CAD build for the part. Positions are in the model's coordinates, mm. A direction names the side the tool comes from. Coordinates: 2 decimals unless noted, no trailing zeros. Loops run counter-clockwise (first coordinate to the right, second up) from the corner with the lowest first, then second, coordinate; pieces in that order, holes last. Notation, with made-up numbers: (12, -22) -> (42, -22) arc R14 ccw to (42, -3) -> close; hole circle Ø11 at (-37.75, 87). An arc over 180 degrees is marked (long way). Answer as CSV lines item,"result". Start each with the question number.
```python
from build123d import *

# Parameters (mm, degrees)
ESBO_O1_R                                   = 9.1
RESSALTO_EXTRUS_O1_DEPTH                    = 3
ESBO_O2_R                                   = 6.7
RESSALTO_EXTRUS_O2_DEPTH                    = 87
FURO_ROSCADO_PARA_CONDU_TE_DE_M4X0_72_D     = 4.2
FURO_ROSCADO_PARA_CONDU_TE_DE_M4X0_72_DEPTH = 22
FURO_ROSCADO_PARA_CONDU_TE_DE_M4X0_72_TIP   = 1.2618073
RESSALTO_EXTRUS_O3_DEPTH                    = 4


with BuildPart() as part:
    # Esboço1 → Ressalto-extrusão1 (new body)
    with BuildSketch(Plane.XY):
        Circle(ESBO_O1_R)
    extrude(amount=-RESSALTO_EXTRUS_O1_DEPTH)

    # Esboço2 → Ressalto-extrusão2 (add)
    with BuildSketch(Plane(origin=(0, 0, -3), x_dir=(-1, 0, 0), z_dir=(0, 0, -1))):
        Circle(ESBO_O2_R)
    extrude(amount=RESSALTO_EXTRUS_O2_DEPTH)

    # Furo roscado para conduíte de M4x0.72
    with Locations(Plane(origin=(0, 0, -90), x_dir=(-1, 0, 0), z_dir=(0, 0, -1))):
        with Locations((0, 0)):
            Hole(FURO_ROSCADO_PARA_CONDU_TE_DE_M4X0_72_D / 2, depth=FURO_ROSCADO_PARA_CONDU_TE_DE_M4X0_72_DEPTH)
            with Locations((0, 0, -(FURO_ROSCADO_PARA_CONDU_TE_DE_M4X0_72_DEPTH + FURO_ROSCADO_PARA_CONDU_TE_DE_M4X0_72_TIP / 2))):  # 118° drill point
                Cone(0, FURO_ROSCADO_PARA_CONDU_TE_DE_M4X0_72_D / 2, FURO_ROSCADO_PARA_CONDU_TE_DE_M4X0_72_TIP, mode=Mode.SUBTRACT)

    # Esboço7 → Ressalto-extrusão3 (add)
    with BuildSketch(Plane(origin=(0, 0, -90), x_dir=(-1, 0, 0), z_dir=(0, 0, -1))):
        with BuildLine():
            Line((-5.37494186, 4), (5.37494186, 4))
            ThreePointArc((5.37494186, 4), (0, 6.7), (-5.37494186, 4))
        make_face()
    extrude(amount=RESSALTO_EXTRUS_O3_DEPTH)


solid = part.part
```
Q1. Probe probe 1 along X at (y, z) = (0, -73.5); probe 2 along Z at (x, y) = (3.5, 6). List the from-to ranges inside material, lowest first. Write a range as from..to.
Q2. Saw through at C-C (z = -41). List the corners of the cut face in (x, y).
Q3. Two-plate mould, pull along Y, no slides. Class faces 4 (the flat face through (0, 5, -94)), 5 (the cylindrical face through (2.003, 0.631, -78.846)), 6 (the flat face through (0, 4, -92)), 7 (the conical face through (-0.35, 0.11, -66.96)): pulls with the +Y half, pulls with the -Y half, needs draft (parallel to the pull), parting line crosses it, or undercut.
Q4. Saw through at A-A (z = -83.5). List the corners of the cut face in (x, y), and give its area (3 significant figures).
Q5. Which spindle directions (+Z, -Z, +X, -X, +Y, -Y) get a long thin tool onto all of the face, cutting with end or side? Do faces 1 (the cylindrical face through (-1.973, -8.884, -1.479)), 2 (the flat face through (-1, -7, -3)), 3 (the flat face through (0.1, -2.5, -90)). Say none if no direction does.
Q6. Pin check, flat tips, straight feed: pin 1 Ø1 at (x, y) = (-3, 4.5) entering from +Z; pin 2 Ø4.5 at (x, z) = (0, -92) entering from -Y; pin 3 Ø3 at (x, z) = (-0.5, -33) entering from +Y; pin 4 Ø9 at (x, y) = (3, -4.5) entering from -Z. Stop position of each tip, or through.
Q7. Saw through at D-D (y = 5.5). List the corners of the cut face in (x, z), and give its area (3 significant figures).
Q8. Saw through at B-B (y = -4.75). List the corners of the cut face in (x, z), and give its area (3 significant figures).
Ans:
1,probe 1,"x = -6.7..-2.1, 2.1..6.7"
1,probe 2,"z = -3..0"
2,outline,"circle Ø13.4 at (0, 0)"
3,face 4,"needs draft"
3,face 5,"undercut"
3,face 6,"pulls with the -Y half"
3,face 7,"undercut"
4,outline,"circle Ø13.4 at (0, 0); hole circle Ø4.2 at (0, 0)"
4,area,"127 mm²"
5,face 1,"+Z, -Z"
5,face 2,"-Z"
5,face 3,"-Z, +X, -X, -Y"
6,pin 1,"stops at z = 0"
6,pin 2,"stops at y = -6.7"
6,pin 3,"stops at y = 6.7"
6,pin 4,"stops at z = -90"
7,outline,"(-7.25, -3) -> (-3.83, -3) -> (-3.83, -94) -> (3.83, -94) -> (3.83, -3) -> (7.25, -3) -> (7.25, 0) -> (-7.25, 0) -> close"
7,area,"740 mm²"
8,outline,"(-7.76, -3) -> (-4.73, -3) -> (-4.73, -90) -> (4.73, -90) -> (4.73, -3) -> (7.76, -3) -> (7.76, 0) -> (-7.76, 0) -> close"
8,area,"869 mm²"
